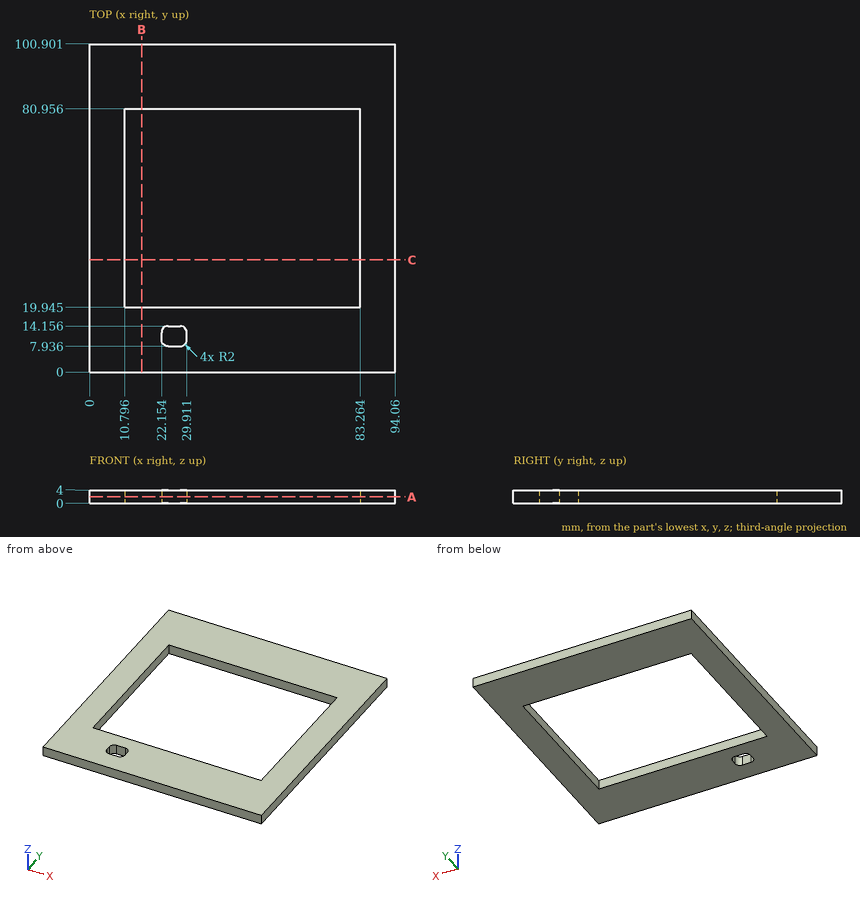
Geometry: see drawing. Coordinates: mm, zero at the bounding-box minimum. Coordinates: 2 decimals unless noted, no trailing zeros. Write each loop counter-clockwise with the first axis right and the second up, starting at its lowest first coordinate (ties: lowest second). Pieces come first, ordered by that corner, then holes. Notation, with made-up numbers: (87, 41) - (135, 41) arc R15 cw to (135, 48) - close; hole circle Ø6 at (0, 58). An arc over 180 degrees is marked (long way). Put each result on its own line as item: value. Start each with the question number.
1) Cut plane A-A (z = 1.9). Return the cut outline in (x, y) (1 decimal).
2) Cut plane C-C (y = 34.5). Return the cut outline in (x, z).
3) Cut plane B-B (x = 16). Return the cut outline in (y, z) (1 decimal).
4) Ray query, L1, parallel to X at y = 21, z = 2.7; L2, parallel to Y at x = 66, z = 2.3 (1 decimal); L3, parallel to Y at x = 28.5, z = 2.4 (1 decimal). Return the intervals inside material, ascending.
Resolved:
1. outline: (0, 0) - (94.1, 0) - (94.1, 100.9) - (0, 100.9) - close; hole (10.8, 19.9) - (83.3, 19.9) - (83.3, 81) - (10.8, 81) - close; hole (22.2, 9.9) arc R2 ccw to (24.2, 7.9) - (27.9, 7.9) arc R2 ccw to (29.9, 9.9) - (29.9, 12.2) arc R2 ccw to (27.9, 14.2) - (24.2, 14.2) arc R2 ccw to (22.2, 12.2) - close
2. outline: (0, 0) - (10.8, 0) - (10.8, 4) - (0, 4) - close; (83.26, 0) - (94.06, 0) - (94.06, 4) - (83.26, 4) - close
3. outline: (0, 0) - (19.9, 0) - (19.9, 4) - (0, 4) - close; (81, 0) - (100.9, 0) - (100.9, 4) - (81, 4) - close
4. L1: x = 0 to 10.8, 83.26 to 94.06
4. L2: y = 0 to 19.9, 81 to 100.9
4. L3: y = 0 to 8, 14.1 to 19.9, 81 to 100.9
